```python
from build123d import *

# Parameters (mm, degrees)
SCHIZZO1_W                   = 40
SCHIZZO1_H                   = 40
ESTRUSIONE_ESTRUSIONE1_DEPTH = 4
ESTRUSIONE_ESTRUSIONE2_DEPTH = 36
SMUSSO1_SIZE                 = 10
FORO_PER_VITE_M4_1_D         = 4.5
FORO_PER_VITE_M4_1_DEPTH     = 9
FORO_PER_VITE_M4_1_TIP       = 1.351936393
FORO_PER_VITE_M4_2_D         = 4.5
FORO_PER_VITE_M4_2_DEPTH     = 9
FORO_PER_VITE_M4_2_TIP       = 1.351936393
FORO_PER_VITE_M4_3_D         = 4.5
FORO_PER_VITE_M4_3_DEPTH     = 9
FORO_PER_VITE_M4_3_TIP       = 1.351936393


with BuildPart() as part:
    # Schizzo1 → Estrusione-Estrusione1 (new body)
    with BuildSketch(Plane(origin=(0, 0, 0), x_dir=(1, 0, 0), z_dir=(0, 1, 0))):
        with Locations((-20, 20)):
            Rectangle(SCHIZZO1_W, SCHIZZO1_H)
    extrude(amount=ESTRUSIONE_ESTRUSIONE1_DEPTH)

    # Schizzo2 → Estrusione-Estrusione2 (add)
    with BuildSketch(Plane(origin=(0, 4, 0), x_dir=(1, 0, 0), z_dir=(0, 1, 0))):
        Polygon((-36, 0), (-40, 0), (-40, 40), (0, 40), (0, 36), (-36, 36), align=None)
    extrude(amount=ESTRUSIONE_ESTRUSIONE2_DEPTH)

    # Smusso1
    smusso1_edges = [part.edges().sort_by_distance(p)[0] for p in [
        (-36, 4, -18),
        (-18, 4, -36),
        (-36, 22, -36),
    ]]
    chamfer(smusso1_edges, length=SMUSSO1_SIZE)

    # Foro per Vite M4-1
    with Locations(Plane(origin=(0, 0, 0), x_dir=(-1, 0, 0), z_dir=(0, -1, 0))):
        with Locations((8.838834765, 19.445436483), (19.445436483, 8.838834765)):
            Hole(FORO_PER_VITE_M4_1_D / 2, depth=FORO_PER_VITE_M4_1_DEPTH)
            with Locations((0, 0, -(FORO_PER_VITE_M4_1_DEPTH + FORO_PER_VITE_M4_1_TIP / 2))):  # 118° drill point
                Cone(0, FORO_PER_VITE_M4_1_D / 2, FORO_PER_VITE_M4_1_TIP, mode=Mode.SUBTRACT)

    # Foro per Vite M4-2
    with Locations(Plane(origin=(0, 0, -40), x_dir=(-1, 0, 0), z_dir=(0, 0, -1))):
        with Locations((8.838834765, 20.554563517), (19.445436483, 31.161165235)):
            Hole(FORO_PER_VITE_M4_2_D / 2, depth=FORO_PER_VITE_M4_2_DEPTH)
            with Locations((0, 0, -(FORO_PER_VITE_M4_2_DEPTH + FORO_PER_VITE_M4_2_TIP / 2))):  # 118° drill point
                Cone(0, FORO_PER_VITE_M4_2_D / 2, FORO_PER_VITE_M4_2_TIP, mode=Mode.SUBTRACT)

    # Foro per Vite M4-3
    with Locations(Plane.ZY.offset(40)):
        with Locations((-19.445436483, 31.161165235), (-8.838834765, 20.554563517)):
            Hole(FORO_PER_VITE_M4_3_D / 2, depth=FORO_PER_VITE_M4_3_DEPTH)
            with Locations((0, 0, -(FORO_PER_VITE_M4_3_DEPTH + FORO_PER_VITE_M4_3_TIP / 2))):  # 118° drill point
                Cone(0, FORO_PER_VITE_M4_3_D / 2, FORO_PER_VITE_M4_3_TIP, mode=Mode.SUBTRACT)


solid = part.part
```
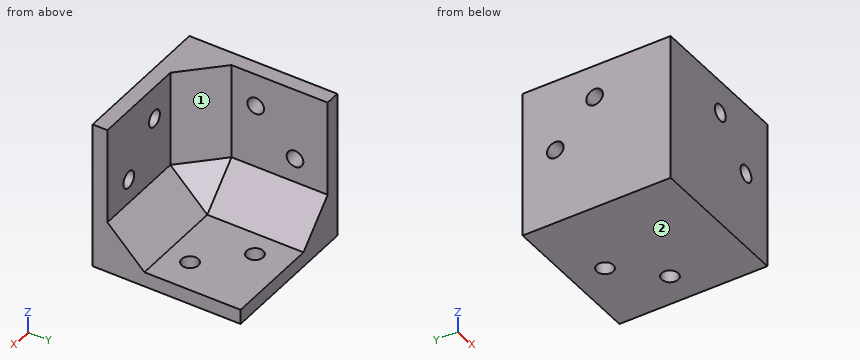
Part model, mm, in its own coordinate system. Face numbers are marked on the shaded views. A direction names the side the tool comes from. Round coordinates to 2 decimals unless told otherwise and drop trailing zeros. Loops run counter-clockwise (first coordinate to the right, second up) from the corner with the lowest first, then second, coordinate; pieces in that order, holes last.
Item 1: Cut at D-D, the plane y = 19. Give the cut face in (x, z).
Item 2: Cut at A-A, the plane y = 24.5. Give the cut face in (x, z).
Item 3: Cut at C-C, the plane x = -9.5. Give the cut face in (y, z).
Item 4: Drill centre lines: line 1 (X direction, y = 34.5, z = -14); line 2 (Y direction, x = -17, z = -7.5). Where is each one in solid material? Low to high.
Item 5: Cut at B-B, the plane z = -34.5. Give the cut face in (x, y).
Item 6: 3-axis set-ups, long thin cutter, end or side, ignore diameter. For the marked faces 1 and 2: which of +Z, -Z, +X, -X, +Y, -Y reach the whole face in a straight line?
Item 7: Drop flat-ended pins along their axis: P1, Ø6, axis at x = -19.45, y = 31.16, coming from the +Z side; P2, Ø8, axis at y = 21, z = -10, coming from the +X side; P3, Ø3, axis at x = -21, z = -22.5, coming from the -Y side; P4, Ø10, axis at x = -28, z = -9, coming from the +Y side. Give the stop position or say it passes through.
A:
1. outline: (-40, -40) - (-10.47, -40) - (-10.47, -36) - (-26, -36) - (-36, -26) - (-36, -10.47) - (-40, -10.47) - close; (-40, -7.21) - (-36, -7.21) - (-36, 0) - (-40, 0) - close; (-7.21, -40) - (0, -40) - (0, -36) - (-7.21, -36) - close
2. outline: (-40, -40) - (0, -40) - (0, -36) - (-26, -36) - (-36, -26) - (-36, 0) - (-40, 0) - close
3. outline: (0, -40) - (18.4, -40) - (18.4, -36) - (14, -36) - (4, -26) - (4, -21.6) - (0, -21.6) - close; (0, -17.29) - (4, -17.29) - (4, 0) - (0, 0) - close; (22.71, -40) - (40, -40) - (40, -36) - (22.71, -36) - close
4. line 1: x = -40 to -36
4. line 2: y = 0 to 4
5. outline: (-40, 0) - (0, 0) - (0, 12.5) - (-26, 12.5) - (-27.5, 14) - (-27.5, 40) - (-40, 40) - close
6. face 1: +Z, +X, +Y
6. face 2: -Z, +X, -X, +Y, -Y
7. P1: stops at z = -36
7. P2: stops at x = -36
7. P3: stops at y = 0
7. P4: stops at y = 11
